Read the model definition and answer for the solid it produces. Units are mm, in the model's axes. Round coordinates to 2 decimals unless told otherwise and drop trailing zeros. Loops run counter-clockwise (first coordinate to the right, second up) from the corner with the lowest first, then second, coordinate; pieces in that order, holes last. Notation, with made-up numbers: (73, -11) - (90, -11) arc R23 cw to (90, 22) - close; hole circle Ø4 at (38.5, 50.25). An arc over 180 degrees is marked (long way). Use CSV: the item, a comma, the result in double quotes. Start each with the question number.
1. Find section A-A (y = 36.5). Give the vertices of the cut face in (x, z).
2. Determine the mould class of faces 1 (the cylindrical face through (-124.88, 5.5, 4.93)), 2 (the cylindrical face through (310, 97.6, 4.9)), 3 (the flat face through (140, 5, 10)) for opening direction Y: +Y half, -Y half, draft (parallel to the pull), parting line (faces both ways), or undercut.
3. Find section D-D (y = -224.5). Give the vertices of the cut face in (x, z), and give its area (3 significant figures).
4. Given pin 1 Ø3 at (x, z) = (-153, 3) entering from +Y; pin 2 Ø6 at (x, z) = (177, 7.5) entering from +Y; pin 3 Ø2 at (x, z) = (86.5, 7.5) entering from +Y, each flat-ended and moving along its own axis, determine where each tip first touches the part or whether it passes through.
5. Find section B-B (x = -90). Give the vertices of the cut face in (y, z).
6. Consider line 1 along X through (y, z) = (-1, 7.5); line 2 along Y through (x, z) = (0, 4); line 3 along X through (y, z) = (-59.5, 3.5). Determine where each line is inside the solid, lowest interval first.
7. Find section C-C (z = 2). State how many separate pieces and enclosed holes the cut face has, and give its area (3 significant figures).
from build123d import *

# Parameters (mm, degrees)
SKETCH1_R           = 325
SKETCH1_R_2         = 125
SKETCH1_R_3         = 6.1
BOSS_EXTRUDE1_DEPTH = 10


with BuildPart() as part:
    # Sketch1 → Boss-Extrude1 (new body)
    with BuildSketch(Plane.XY):
        Circle(SKETCH1_R)
        Circle(SKETCH1_R_2, mode=Mode.SUBTRACT)
        with Locations((0, 150)):
            Circle(SKETCH1_R_3, mode=Mode.SUBTRACT)
        with Locations((57.402514855, 138.581929877)):
            Circle(SKETCH1_R_3, mode=Mode.SUBTRACT)
        with Locations((106.066017178, 106.066017178)):
            Circle(SKETCH1_R_3, mode=Mode.SUBTRACT)
        with Locations((138.581929877, 57.402514855)):
            Circle(SKETCH1_R_3, mode=Mode.SUBTRACT)
        with Locations((150, 0)):
            Circle(SKETCH1_R_3, mode=Mode.SUBTRACT)
        with Locations((138.581929877, -57.402514855)):
            Circle(SKETCH1_R_3, mode=Mode.SUBTRACT)
        with Locations((106.066017178, -106.066017178)):
            Circle(SKETCH1_R_3, mode=Mode.SUBTRACT)
        with Locations((57.402514855, -138.581929877)):
            Circle(SKETCH1_R_3, mode=Mode.SUBTRACT)
        with Locations((0, -150)):
            Circle(SKETCH1_R_3, mode=Mode.SUBTRACT)
        with Locations((-57.402514855, -138.581929877)):
            Circle(SKETCH1_R_3, mode=Mode.SUBTRACT)
        with Locations((-106.066017178, -106.066017178)):
            Circle(SKETCH1_R_3, mode=Mode.SUBTRACT)
        with Locations((-138.581929877, -57.402514855)):
            Circle(SKETCH1_R_3, mode=Mode.SUBTRACT)
        with Locations((-150, 0)):
            Circle(SKETCH1_R_3, mode=Mode.SUBTRACT)
        with Locations((-138.581929877, 57.402514855)):
            Circle(SKETCH1_R_3, mode=Mode.SUBTRACT)
        with Locations((-106.066017178, 106.066017178)):
            Circle(SKETCH1_R_3, mode=Mode.SUBTRACT)
        with Locations((-57.402514855, 138.581929877)):
            Circle(SKETCH1_R_3, mode=Mode.SUBTRACT)
    extrude(amount=BOSS_EXTRUDE1_DEPTH)


solid = part.part
Filled sheet:
1,outline,"(-322.94, 0) - (-119.55, 0) - (-119.55, 10) - (-322.94, 10) - close; (119.55, 0) - (322.94, 0) - (322.94, 10) - (119.55, 10) - close"
2,face 1,"undercut"
2,face 2,"parting line"
2,face 3,"draft"
3,outline,"(-235, 0) - (235, 0) - (235, 10) - (-235, 10) - close"
3,area,"4,700 mm²"
4,pin 1,"stops at y = 287.53"
4,pin 2,"stops at y = 274.5"
4,pin 3,"stops at y = 313.55"
5,outline,"(-312.29, 0) - (-86.75, 0) - (-86.75, 10) - (-312.29, 10) - close; (86.75, 0) - (312.29, 0) - (312.29, 10) - (86.75, 10) - close"
6,line 1,"x = -325 to -156.02, -143.98 to -125, 125 to 143.98, 156.02 to 325"
6,line 2,"y = -325 to -156.1, -143.9 to -125, 125 to 143.9, 156.1 to 325"
6,line 3,"x = -319.51 to -144.31, -132.85 to -109.93, 109.93 to 132.85, 144.31 to 319.51"
7,separate pieces,"1"
7,enclosed holes,"17"
7,area,"281,000 mm²"
